Autodesk Inventor part; units mm, degrees
ref_plane "YZ Plane" through (0, 0, 0) normal (1, 0, 0) x (0, 1, 0)
ref_plane "XZ Plane" through (0, 0, 0) normal (0, 1, 0) x (-1, 0, 0)
ref_plane "XY Plane" through (0, 0, 0) normal (0, 0, 1) x (1, 0, 0)
sketch "スケッチ1" plane through (0, 0, 0) normal (0, 0, 1) x (0, 1, 0)
  circle A0 centre (12, 0) radius 4 construction
  arc A1 (2, 0) -> (6.1183, -8.0874) centre (12, 0) ccw
  arc A2 (6.8885, -8.8489) -> (6.1183, -8.0874) centre (4, -11) ccw
  line L0 (-23.25, 12.25) -> (-23.25, -12.25) construction
  line L1 (-23.25, -12.25) -> (-21.25, -14.25) construction
  line L2 (-21.25, -14.25) -> (21.25, -14.25) construction
  line L3 (0, 0) -> (2, 0)
  line L4 (0, 0) -> (-23.25, 0)
  line L5 (-23.25, 0) -> (-23.25, -12.25)
  line L6 (-23.25, -12.25) -> (-21.25, -14.25)
  line L7 (-0.4772, -29.5258) -> (4.929, -39.7419)
  line L8 (6.8885, -8.8489) -> (13.2614, -17.4062)
  line L9 (13.2614, -17.4062) -> (19.4413, -33.0628)
  line L10 (2, 0) -> (12, 0) construction
  circle A3 centre (4, -11) radius 1.25 construction
  arc A4 (4.929, -39.7419) -> (19.4413, -33.0628) centre (12, -36) ccw
  circle A5 centre (-20, -11) radius 1.25 construction
  line L11 (12, 0) -> (12, -36) construction
  line L12 (-21.25, -14.25) -> (-0.4772, -14.25)
  line L13 (-0.4772, -29.5258) -> (-0.4772, -14.25)
  dimension "d0" = 10
  dimension "d3" = 36
  dimension "d4" = 8
extrude "押し出し1" add sketch "スケッチ1" along normal blind 2
hole "穴1" at (36, 12, 0) direction (0, 0, 1) diameter 3 end through all
hole "穴2" at (11, 4, 0) at (11, -20, 0) direction (0, 0, 1) diameter 2.5 end through all
properties part number "HIP_TOPFRAME2"
Model file for the job. Use its own axes, mm. A direction names the side the tool comes from. Coordinates: 2 decimals unless noted, no trailing zeros. Loops run counter-clockwise (first coordinate to the right, second up) from the corner with the lowest first, then second, coordinate; pieces in that order, holes last. Notation, with made-up numbers: (28.25, 35.5) -> (82.25, 35.5) arc R22 cw to (82.25, 45.5) -> close; hole circle Ø8 at (44.25, 64.25). An arc over 180 degrees is marked (long way). Use one line per item in the form item = value. Start each with the question number.
(1) Cut at D-D on x = 36. Give the cut face in (y, z), and give its area (3 significant figures).
(2) Probe probe 1 along X at (y, z) = (-20, 0.95); probe 2 along Y at (x, z) = (11, 1); probe 3 along X at (y, z) = (-6, 0.95). List the from-to ranges inside material, lowest first. Write a range as from..to.
(3) Cut at C-C on x = 10.5. Give the cut face in (y, z), and give its area (3 significant figures).
(4) Tool access for faces 1 (the flat face through (22, -0.477, 1)), 2 (the cylindrical face through (4.6, 3.12, 0.99)): list every direction of +Z, -Z, +X, -X, +Y, -Y with a clear straight run to the whole face (end or side of a thin tool).
(5) Flat gauge pins, fed straight in: pin 1 (5 mm diameter, centred on x = 36, y = 12, fed in from -Z); pin 2 (12 mm diameter, centred on x = 20.5, y = -9.5, fed in from +Z); pin 3 (1 mm diameter, centred on y = 8, z = 0.5, fed in from -X). Where does each tip first touch, or does it go through?
(6) Cut at B-B on z = 0.65. Give the cut face in (x, y).
(7) Cut at A-A on y = -20. Give the cut face in (x, z).
(8) Pull direction X, two halves, no side cores. Call faces 3 (the cylindrical face through (10.62, -18.81, 1.01)), 4 (the cylindrical face through (9.946, 4.672, 1.014)), 5 (the cylindrical face through (43.195, 15.498, 0.986)), 6 (the flat face through (0, -11, 1)): pulls with the +X half, pulls with the -X half, needs draft (parallel to the pull), parting line crosses it, or undercut.
Values:
q1.outline = (2.95, 0) -> (10.5, 0) -> (10.5, 2) -> (2.95, 2) -> close; (13.5, 0) -> (20, 0) -> (20, 2) -> (13.5, 2) -> close
q1.area = 28.1 mm2
q2.probe_1 = 0..9.75, 12.25..14.25
q2.probe_2 = -23.25..-21.25, -18.75..2.75, 5.25..8.49
q2.probe_3 = 0..14.25
q3.outline = (-23.25, 0) -> (-21.15, 0) -> (-21.15, 2) -> (-23.25, 2) -> close; (-18.85, 0) -> (2.85, 0) -> (2.85, 2) -> (-18.85, 2) -> close; (5.15, 0) -> (8.12, 0) -> (8.12, 2) -> (5.15, 2) -> close
q3.area = 53.6 mm2
q4.face_1 = +Z, -Z, +X, -Y
q4.face_2 = +Z, -Z, -X, +Y
q5.pin_1 = 0
q5.pin_2 = through
q5.pin_3 = 9.67
q6.outline = (0, -23.25) -> (12.25, -23.25) -> (14.25, -21.25) -> (14.25, -0.48) -> (29.53, -0.48) -> (39.74, 4.93) arc R8 ccw to (33.06, 19.44) -> (17.41, 13.26) -> (8.85, 6.89) arc R3.6 ccw to (8.09, 6.12) arc R10 cw to (0, 2) -> close; hole circle Ø2.5 at (11, -20); hole circle Ø2.5 at (11, 4); hole circle Ø3 at (36, 12)
q7.outline = (0, 0) -> (9.75, 0) -> (9.75, 2) -> (0, 2) -> close; (12.25, 0) -> (14.25, 0) -> (14.25, 2) -> (12.25, 2) -> close
q8.face_3 = undercut
q8.face_4 = undercut
q8.face_5 = parting line crosses it
q8.face_6 = pulls with the -X half
